Autodesk Inventor part; units mm, degrees
ref_plane "YZ Plane" through (0, 0, 0) normal (1, 0, 0) x (0, 1, 0)
ref_plane "XZ Plane" through (0, 0, 0) normal (0, 1, 0) x (-1, 0, 0)
ref_plane "XY Plane" through (0, 0, 0) normal (0, 0, 1) x (1, 0, 0)
sketch "草圖1" plane through (0, 0, 0) normal (0, 1, 0) x (-1, 0, 0)
  line L0 (85, 85) -> (-85, 85)
  line L1 (-85, 85) -> (-85, -85)
  line L2 (-85, -85) -> (85, -85)
  line L3 (85, -85) -> (85, 85)
  line L4 (85, 85) -> (-85, -85) construction
  line L5 (-85, 85) -> (85, -85) construction
  point P0 (0, 0)
  dimension "d0" = 170
  dimension "d1" = 170
extrude "擠出1" add sketch "草圖1" along normal blind 9
sketch "草圖2" plane through (0, 9, 0) normal (0, 1, 0) x (1, 0, 0)
  line L0 (-85, 85) -> (-85, -85)
  line L1 (-85, -85) -> (-65, -85)
  line L2 (-65, -85) -> (-65, -65)
  line L3 (-65, -65) -> (-85, -65)
  line L4 (-85, -65) -> (-85, -85)
  point P0 (0, 0)
  dimension "d4" = 20
  dimension "d5" = 20
extrude "擠出2" cut sketch "草圖2" against normal through all
pattern_circular "環形陣列1" count 4 over 360 about axis through (0, -10, 0) along (0, 1, 0) of "擠出2"
sketch "草圖5" plane through (0, 9, 0) normal (0, 1, 0) x (1, 0, 0)
  point P0 (0, 0)
  point P1 (0, 0)
hole "孔3" at (0, 9, 0) direction (0, -1, 0) diameter 11 end through all
sketch "草圖6" plane through (0, 9, 0) normal (0, 1, 0) x (1, 0, 0)
  point P0 (0, 0)
  point P1 (-15.5, 0)
  point P2 (15.5, 0)
  dimension "d36" = 31
  dimension "d37" = 15.5
hole "孔4" at (-15.5, 9, 0) at (15.5, 9, 0) direction (0, -1, 0) diameter 5 end through all
equation "\"d0\" = d1"
properties part number "上部3分木板中板" material "松木、赤松"
CAD build for the part. Positions are in the model's coordinates, mm. A direction names the side the tool comes from. Give positions to 0.01 mm unless a question says otherwise; leave off trailing zeros. Write each loop counter-clockwise with the first axis right and the second up, starting at its lowest first coordinate (ties: lowest second). Pieces come first, ordered by that corner, then holes. Notation, with made-up numbers: M -4.75,43 L 28.25,43 A14 cw 28.25,70 Z; hole C 83,12.25 d3. An arc over 180 degrees is marked long. Return JSON: item names as keys, results as strings. Group by question number.
(1) 3-axis set-ups, long thin cutter, end or side, ignore diameter. For faces 1 (the face through (75, 5, 65)), 2 (the face through (-65, 5, -75)), 3 (the face through (-75, 5, 65)), 4 (the face through (65, 5, -75)), 5 (the face through (85, 4, 1)): which of +Z, -Z, +X, -X, +Y, -Y reach the whole face in a straight line?
(2) Band-saw the part on C-C (y = 6.75). Give the cut face in (x, z).
(3) Band-saw the part on D-D (z = -70). Give the cut face in (x, y).
(4) Drill centre lines: L1, parallel to X at y = 6, z = 0; L2, parallel to Z at x = 0, y = 6.5; L3, parallel to Z at x = -15.5, y = 2.5. Where is each one in solid material? Low to high. Write a range as [from, to].
(5) Band-saw the part on B-B (z = 0). Give the cut face in (x, y).
(6) Band-saw the part on A-A (x = 0). Give the cut face in (y, z).
(7) Mould opens along X. For faces 6 (the face through (-13.06, 4.44, -0.54)), 7 (the face through (65, 5, 75)), 8 (the face through (20, 0, 1)) say: pulls with the +X half, pulls with the -X half, needs draft (parallel to the pull), parting line crosses it, or undercut.
(8) Flat gauge pin, fed straight in: pin 1 Ø4.5 at (y, z) = (2.5, -78.5) entering from -X. Where does the tip first touch, or does it go through?
Entries:
{
 "1": {"face 1": "+Z, +X, +Y, -Y", "face 2": "-Z, -X, +Y, -Y", "face 3": "+Z, -X, +Y, -Y", "face 4": "-Z, +X, +Y, -Y", "face 5": "+Z, -Z, +X, +Y, -Y"},
 "2": {"outline": "M -85,-65 L -65,-65 L -65,-85 L 65,-85 L 65,-65 L 85,-65 L 85,65 L 65,65 L 65,85 L -65,85 L -65,65 L -85,65 Z; hole C -15.5,0 d5; hole C 0,0 d11; hole C 15.5,0 d5"},
 "3": {"outline": "M -65,0 L 65,0 L 65,9 L -65,9 Z"},
 "4": {"L1": "x = [-85, -18], [-13, -5.5], [5.5, 13], [18, 85]", "L2": "z = [-85, -5.5], [5.5, 85]", "L3": "z = [-85, -2.5], [2.5, 85]"},
 "5": {"outline": "M -85,0 L -18,0 L -18,9 L -85,9 Z; M -13,0 L -5.5,0 L -5.5,9 L -13,9 Z; M 5.5,0 L 13,0 L 13,9 L 5.5,9 Z; M 18,0 L 85,0 L 85,9 L 18,9 Z"},
 "6": {"outline": "M 0,-85 L 9,-85 L 9,-5.5 L 0,-5.5 Z; M 0,5.5 L 9,5.5 L 9,85 L 0,85 Z"},
 "7": {"face 6": "undercut", "face 7": "pulls with the +X half", "face 8": "needs draft"},
 "8": {"pin 1": "stops at x = -65"}
}
